Geometry check sheet. Reference: the model listing, model coordinates, mm. Give positions to 0.01 mm unless a question says otherwise; leave off trailing zeros. Order: outer loops, then holes, each group sorted by start corner. A loop starts at its lowest first (then second) coordinate and runs counter-clockwise, first axis right, second up.
```python
from build123d import *

# Parameters (mm, degrees)
SKETCH1_R                              = 17
OUTER_BARREL_CREATION_DEPTH            = 540
SKETCH4_W                              = 100
SKETCH4_H                              = 19
SCREW_INTAKE_EXTRUDE_DEPTH             = 18
SCREW_INTAKE_EXTRUDE_DEPTH_BACK        = 18
SKETCH6_W                              = 120
SKETCH6_H                              = 5
PARALLEL_FIN_SIDE_EXTRUSION_DEPTH      = 19
PARALLEL_FIN_SIDE_EXTRUSION_DEPTH_BACK = 19
SKETCH7_W                              = 3.734431396
SKETCH7_H                              = 120
PARALLEL_FIN_HEIGHT_SIDE_1_DEPTH       = 26
SKETCH8_W                              = 3.734431396
SKETCH8_H                              = 120
PARALLEL_FIN_HEIGHT_SIDE_2_DEPTH       = 26
SKETCH9_R                              = 3
PARALLEL_FIN_DETAILS_DEPTH             = 39
SKETCH2_R                              = 13
INNER_BARREL_EXTRUSION_DEPTH           = 541
SKETCH11_W                             = 100
SKETCH11_H                             = 4
BOSS_EXTRUDE6_DEPTH                    = 26
SKETCH12_R                             = 1.5
CUT_EXTRUDE5_DEPTH                     = 4
SKETCH13_R                             = 27.099065824
SKETCH13_R_2                           = 16
CUT_EXTRUDE8_DEPTH                     = 23


with BuildPart() as part:
    # Sketch1 → Outer Barrel Creation (new body)
    with BuildSketch(Plane.XY):
        Circle(SKETCH1_R)
    extrude(amount=-OUTER_BARREL_CREATION_DEPTH)

    # Sketch4 → Screw Intake Extrude (cut, two sides)
    with BuildSketch(Plane(origin=(0, 0, 0), x_dir=(0, 0, -1), z_dir=(1, 0, 0))) as screw_intake_extrude_sk:
        with Locations((125, -7.5)):
            Rectangle(SKETCH4_W, SKETCH4_H)
    extrude(amount=SCREW_INTAKE_EXTRUDE_DEPTH, mode=Mode.SUBTRACT)
    extrude(screw_intake_extrude_sk.sketch, amount=-SCREW_INTAKE_EXTRUDE_DEPTH_BACK, mode=Mode.SUBTRACT)

    # Sketch6 → Parallel Fin Side Extrusion (add, two sides)
    with BuildSketch(Plane(origin=(0, 0, 0), x_dir=(0, 0, -1), z_dir=(1, 0, 0))) as parallel_fin_side_extrusion_sk:
        with Locations((125, 4.980803112)):
            Rectangle(SKETCH6_W, SKETCH6_H)
    extrude(amount=PARALLEL_FIN_SIDE_EXTRUSION_DEPTH)
    extrude(parallel_fin_side_extrusion_sk.sketch, amount=-PARALLEL_FIN_SIDE_EXTRUSION_DEPTH_BACK)

    # Sketch7 → Parallel Fin Height Side 1 (add)
    with BuildSketch(Plane(origin=(0, 7.480803112, 0), x_dir=(1, 0, 0), z_dir=(0, 1, 0))):
        with Locations((17.132784302, 125)):
            Rectangle(SKETCH7_W, SKETCH7_H)
    extrude(amount=PARALLEL_FIN_HEIGHT_SIDE_1_DEPTH)

    # Sketch8 → Parallel Fin Height Side 2 (add)
    with BuildSketch(Plane(origin=(0, 7.480803112, 0), x_dir=(1, 0, 0), z_dir=(0, 1, 0))):
        with Locations((-17.132784302, 125)):
            Rectangle(SKETCH8_W, SKETCH8_H)
    extrude(amount=PARALLEL_FIN_HEIGHT_SIDE_2_DEPTH)

    # Sketch9 → Parallel Fin Details (cut, through all)
    with BuildSketch(Plane.ZY.offset(19)):
        with Locations((-175, 23.480803112)):
            Circle(SKETCH9_R)
        with Locations((-75, 23.480803112)):
            Circle(SKETCH9_R)
        Polygon((-180, 33.480803112), (-185, 28.480803112), (-185, 33.480803112), align=None)
        Polygon((-70, 33.480803112), (-65, 28.480803112), (-65, 33.480803112), align=None)
    extrude(amount=-PARALLEL_FIN_DETAILS_DEPTH, mode=Mode.SUBTRACT)

    # Sketch2 → Inner Barrel Extrusion (cut, through all)
    with BuildSketch(Plane.XY):
        Circle(SKETCH2_R)
    extrude(amount=-INNER_BARREL_EXTRUSION_DEPTH, mode=Mode.SUBTRACT)

    # Sketch11 → Boss-Extrude6 (add)
    with BuildSketch(Plane(origin=(0, 0, 0), x_dir=(0, 0, -1), z_dir=(0.707106781, 0.707106781, 0))):
        with Locations((125, 14.15826017)):
            Rectangle(SKETCH11_W, SKETCH11_H)
    boss_extrude6 = extrude(amount=-BOSS_EXTRUDE6_DEPTH)

    # Sketch12 → Cut-Extrude5 (cut)
    with BuildSketch(Plane(origin=(-11.425615339, 11.425615339, 0), x_dir=(0, 0, 1), z_dir=(-0.707106781, 0.707106781, 0))):
        with Locations((-162, -16)):
            Circle(SKETCH12_R)
        with Locations((-88, -16)):
            Circle(SKETCH12_R)
        Polygon((-175, -7.468207578), (-166, -26), (-175, -26), align=None)
        Polygon((-75, -6.46439117), (-75, -26), (-84, -26), align=None)
    cut_extrude5 = extrude(amount=-CUT_EXTRUDE5_DEPTH, mode=Mode.SUBTRACT)

    # Mirror2: Boss-Extrude6, Cut-Extrude5 across plane
    add(boss_extrude6.mirror(Plane(origin=(0, 0, 0), x_dir=(0, 0, 1), z_dir=(1, 0, 0))))
    add(cut_extrude5.mirror(Plane(origin=(0, 0, 0), x_dir=(0, 0, 1), z_dir=(1, 0, 0))), mode=Mode.SUBTRACT)

    # Sketch13 → Cut-Extrude8 (cut)
    with BuildSketch(Plane(origin=(0, 0, -540), x_dir=(-1, 0, 0), z_dir=(0, 0, -1))):
        Circle(SKETCH13_R)
        Circle(SKETCH13_R_2, mode=Mode.SUBTRACT)
    extrude(amount=-CUT_EXTRUDE8_DEPTH, mode=Mode.SUBTRACT)


solid = part.part
```
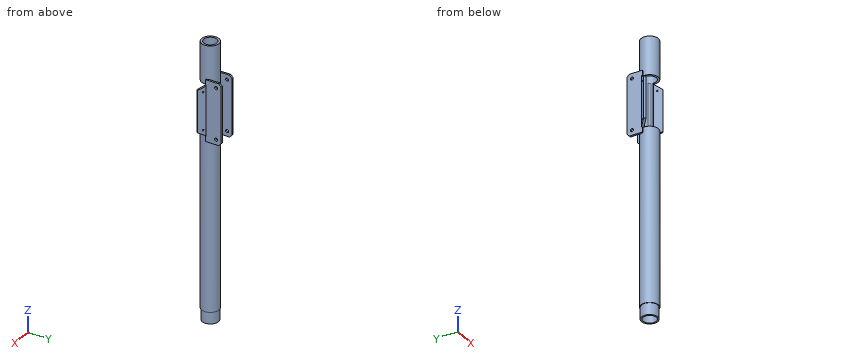
Q1. Gauge pin test, flat ends, axial feed: P1, Ø2.5, axis at x = -18.5, z = -180, coming from the -Y side; P2, Ø1.9, axis at x = -13.5, z = -147, coming from the -Y side; P3, Ø3, axis at y = 6, z = -410, coming from the -X side; P4, Ø5, axis at y = 23.48, z = -75, coming from the -X side (3 decimals). Record the tip position at first contact, or that the pin passes through.
Q2. Cross-section at A-A, the plane x = 0. Record the boundary of the cut face in (y, z).
Q3. Cross-section at C-C, the plane z = -454.5. Record the boundary of the cut face in (x, y).
Q4. Thickness scan on L1, parallel to Z at x = 14.5, y = -6; L2, parallel to X at y = -1, z = -419; L3, parallel to X at y = 25.5, z = -150. Record the ranges inside material, lowest first.
Q5. Cross-section at B-B, the plane z = -148. Record the boundary of the cut face in (x, y), and give its area (3 significant figures).
Answers follow:
1. P1: stops at y = 2.48
1. P2: stops at y = 2
1. P3: stops at x = -16.39
1. P4: passes through
2. outline: (-17, -517) - (-16, -517) - (-16, -540) - (-13, -540) - (-13, -175) - (-17, -175) - close; (-17, -75) - (-13, -75) - (-13, 0) - (-17, 0) - close; (13, -540) - (16, -540) - (16, -517) - (17, -517) - (17, 0) - (13, 0) - close
3. outline: circle Ø34 at (0, 0); hole circle Ø26 at (0, 0)
4. L1: z = -540 to -175, -75 to 0
4. L2: x = -16.97 to -12.96, 12.96 to 16.97
4. L3: x = -19 to -15.27, 15.27 to 19
5. outline: (-29.81, -6.96) - (-26.98, -9.79) - (-15.19, 2) - (-12.85, 2) arc R13 cw to (-11.85, 5.34) - (-8.6, 8.6) - (-9.19, 9.19) arc R13 cw to (9.19, 9.19) - (8.6, 8.6) - (11.85, 5.34) arc R13 cw to (12.85, 2) - (15.19, 2) - (26.98, -9.79) - (29.81, -6.96) - (19, 3.85) - (19, 33.48) - (15.27, 33.48) - (15.27, 7.59) - (15.16, 7.69) arc R17 ccw to (-15.16, 7.69) - (-15.27, 7.59) - (-15.27, 33.48) - (-19, 33.48) - (-19, 3.85) - close
5. area: 523 mm2
